```python
from build123d import *

# Parameters (mm, degrees)
F0_W     = 152.4
F0_H     = 38.1
F0_R     = 6.35
F1_DEPTH = 12.7
F2_DEPTH = 12.7


with BuildPart() as f1:
    # F0 (on Front) → F1 (new body)
    with BuildSketch(Plane.XZ):
        with Locations((-0.336899, 18.955347)):
            Rectangle(F0_W, F0_H)
        with Locations((-63.836899, 18.955347)):
            Circle(F0_R, mode=Mode.SUBTRACT)
        with Locations((63.163101, 18.955347)):
            Circle(F0_R, mode=Mode.SUBTRACT)
    extrude(amount=F1_DEPTH)

    # F0 (on Front) → F2 (join)
    with BuildSketch(Plane.XZ):
        Polygon((75.863101, -0.094653), (-76.536899, -0.094653), (-76.536899, -38.194653), (-0.336899, -38.194653), (75.863101, -38.194653), align=None)
        with Locations((-63.836899, -19.144653)):
            Circle(F0_R, mode=Mode.SUBTRACT)
        with Locations((63.163101, -19.144653)):
            Circle(F0_R, mode=Mode.SUBTRACT)
    extrude(amount=F2_DEPTH)


solid = f1.part
```
Model file for the job. Use its own axes, mm. Round coordinates to 2 decimals unless told otherwise and drop trailing zeros. Write each loop counter-clockwise with the first axis right and the second up, starting at its lowest first coordinate (ties: lowest second). Pieces come first, ordered by that corner, then holes. Notation, with made-up numbers: (-20.75, -24.75) -> (7.25, -24.75) arc R25 ccw to (7.25, -1.75) -> close; hole circle Ø10 at (-5.75, 32.5). An arc over 180 degrees is marked (long way). Answer as CSV lines item,"result".
1. Mould opens along X. For faces 1 (the face through (-76.537, -6, 0)), 2 (the face through (-1, -6, -38.195)), 3 (the face through (-57.971, -6.261, 16.523)), 4 (the face through (75.863, -6, -1)) say: +X half, -X half, draft (parallel to the pull), parting line (faces both ways), or undercut.
Resolved:
face 1,"-X half"
face 2,"draft"
face 3,"undercut"
face 4,"+X half"
2. Drill centre lines: line 1 (X direction, y = -1.5, z = -18.5); line 2 (X direction, y = -1.5, z = 24); line 3 (Z direction, x = 59, y = -5). Where is each one in solid material? Low to high.
Resolved:
line 1,"-76.54 to -70.15, -57.52 to 56.85, 69.48 to 75.86"
line 2,"-76.54 to -67.69, -59.98 to 59.31, 67.02 to 75.86"
line 3,"-38.19 to -23.94, -14.35 to 14.16, 23.75 to 38.01"
3. Slice it at C-C, the plane z = 15.5. List the corners of the cut face in (x, y).
Resolved:
outline,"(-76.54, -12.7) -> (-69.16, -12.7) -> (-69.16, 0) -> (-76.54, 0) -> close; (-58.51, -12.7) -> (57.84, -12.7) -> (57.84, 0) -> (-58.51, 0) -> close; (68.49, -12.7) -> (75.86, -12.7) -> (75.86, 0) -> (68.49, 0) -> close"
4. Slice it at A-A, the plane x = -59. List the corners of the cut face in (y, z).
Resolved:
outline,"(-12.7, -38.19) -> (0, -38.19) -> (0, -23.26) -> (-12.7, -23.26) -> close; (-12.7, -15.03) -> (0, -15.03) -> (0, 14.84) -> (-12.7, 14.84) -> close; (-12.7, 23.07) -> (0, 23.07) -> (0, 38.01) -> (-12.7, 38.01) -> close"
5. Slice it at B-B, the plane y = -8. List the corners of the cut face in (x, z).
Resolved:
outline,"(-76.54, -38.19) -> (75.86, -38.19) -> (75.86, 38.01) -> (-76.54, 38.01) -> close; hole circle Ø12.7 at (-63.84, -19.14); hole circle Ø12.7 at (-63.84, 18.96); hole circle Ø12.7 at (63.16, -19.14); hole circle Ø12.7 at (63.16, 18.96)"
